from build123d import *

# Parameters (mm, degrees)
SKETCH1_R            = 7
BOSS_EXTRUDE1_DEPTH  = 8.9
CUT_EXTRUDE1_REACH   = 42.255
SKETCH6_R            = 1.3
CIRPATTERN1_COUNT    = 4
CUT_EXTRUDE2_REACH   = 42.255
SKETCH7_R            = 1.3
CUT_EXTRUDE3_DEPTH   = 5
SKETCH10_W           = 10
SKETCH10_H           = 8.9
BOSS_EXTRUDE2_DEPTH  = 10
SKETCH11_W           = 10
SKETCH11_H           = 10
BOSS_EXTRUDE3_DEPTH  = 20.4
SKETCH12_W           = 7.6
SKETCH12_H           = 7.6
CUT_EXTRUDE4_DEPTH   = 5
CUT_EXTRUDE5_REACH   = 54.931
SKETCH13_R           = 1.7
FILLET1_R            = 1
FILLET1_OF_MIRROR2_R = 1
MIRROR3_START        = -20.4
MIRROR3_OUTLINE_R    = 1.7
MIRROR3_DEPTH        = 24.3
MIRROR3_START_2      = 3.9
MIRROR3_2_DEPTH      = 5
FILLET2_R            = 0.5


# Read off the part's stored shape, not the designer's step: Mirror3
with BuildPart() as part:
    # Sketch1 → Boss-Extrude1 (new body)
    with BuildSketch(Plane(origin=(0, 0, 0), x_dir=(1, 0, 0), z_dir=(0, 1, 0))):
        with BuildLine():
            Line((-25, -28.5), (17, -28.5))
            ThreePointArc((17, -28.5), (18.414213562, -27.914213562), (19, -26.5))
            Line((19, -26.5), (19, 26.5))
            ThreePointArc((19, 26.5), (18.414213562, 27.914213562), (17, 28.5))
            Line((17, 28.5), (-25, 28.5))
            ThreePointArc((-25, 28.5), (-26.414213562, 27.914213562), (-27, 26.5))
            Line((-27, 26.5), (-27, -26.5))
            ThreePointArc((-27, -26.5), (-26.414213562, -27.914213562), (-25, -28.5))
        make_face()
        with Locations(Location((0, 0, 0), (0, 0, 270))):
            Circle(SKETCH1_R, mode=Mode.SUBTRACT)
    extrude(amount=BOSS_EXTRUDE1_DEPTH)

    # Sketch6 → Cut-Extrude1 (cut, up to next)
    with BuildSketch(Plane(origin=(0, 8.9, 0), x_dir=(1, 0, 0), z_dir=(0, 1, 0)), mode=Mode.PRIVATE) as cut_extrude1_sk1:
        with Locations(Location((-6.703372286, -6.703372286, 0), (0, 0, 270))):
            Circle(SKETCH6_R)
    cut_extrude1_tool1 = extrude(cut_extrude1_sk1.sketch, amount=-CUT_EXTRUDE1_REACH, mode=Mode.PRIVATE) & part.part
    cut_extrude1 = cut_extrude1_tool1.solids().sort_by_distance((-6.703372, 8.9, 6.703372))[0]
    add(cut_extrude1, mode=Mode.SUBTRACT)

    # CirPattern1: Cut-Extrude1 ×4 about axis
    cirpattern1_axis = Axis((0, 0, 0), (0, 1, 0))
    for i in range(1, CIRPATTERN1_COUNT):
        add(cut_extrude1.rotate(cirpattern1_axis, i * 360 / CIRPATTERN1_COUNT), mode=Mode.SUBTRACT)

    # Sketch7 → Cut-Extrude2 (cut, up to next)
    with BuildSketch(Plane(origin=(0, 8.9, 0), x_dir=(1, 0, 0), z_dir=(0, 1, 0)), mode=Mode.PRIVATE) as cut_extrude2_sk1:
        with Locations(Location((-23.5, -20, 0), (0, 0, 270))):
            Circle(SKETCH7_R)
    cut_extrude2_tool1 = extrude(cut_extrude2_sk1.sketch, amount=-CUT_EXTRUDE2_REACH, mode=Mode.PRIVATE) & part.part
    # Sketch7 → Cut-Extrude2 (cut, up to next)
    with BuildSketch(Plane(origin=(0, 8.9, 0), x_dir=(1, 0, 0), z_dir=(0, 1, 0)), mode=Mode.PRIVATE) as cut_extrude2_sk2:
        with Locations(Location((-23.5, 20, 0), (0, 0, 270))):
            Circle(SKETCH7_R)
    cut_extrude2_tool2 = extrude(cut_extrude2_sk2.sketch, amount=-CUT_EXTRUDE2_REACH, mode=Mode.PRIVATE) & part.part
    # Sketch7 → Cut-Extrude2 (cut, up to next)
    with BuildSketch(Plane(origin=(0, 8.9, 0), x_dir=(1, 0, 0), z_dir=(0, 1, 0)), mode=Mode.PRIVATE) as cut_extrude2_sk3:
        with Locations(Location((14.8, -20, 0), (0, 0, 270))):
            Circle(SKETCH7_R)
    cut_extrude2_tool3 = extrude(cut_extrude2_sk3.sketch, amount=-CUT_EXTRUDE2_REACH, mode=Mode.PRIVATE) & part.part
    # Sketch7 → Cut-Extrude2 (cut, up to next)
    with BuildSketch(Plane(origin=(0, 8.9, 0), x_dir=(1, 0, 0), z_dir=(0, 1, 0)), mode=Mode.PRIVATE) as cut_extrude2_sk4:
        with Locations(Location((14.8, 20, 0), (0, 0, 270))):
            Circle(SKETCH7_R)
    cut_extrude2_tool4 = extrude(cut_extrude2_sk4.sketch, amount=-CUT_EXTRUDE2_REACH, mode=Mode.PRIVATE) & part.part
    add(cut_extrude2_tool1.solids().sort_by_distance((-23.5, 8.9, 20))[0], mode=Mode.SUBTRACT)
    add(cut_extrude2_tool2.solids().sort_by_distance((-23.5, 8.9, -20))[0], mode=Mode.SUBTRACT)
    add(cut_extrude2_tool3.solids().sort_by_distance((14.8, 8.9, 20))[0], mode=Mode.SUBTRACT)
    add(cut_extrude2_tool4.solids().sort_by_distance((14.8, 8.9, -20))[0], mode=Mode.SUBTRACT)

    # Sketch8 → Cut-Extrude3 (cut)
    with BuildSketch(Plane(origin=(0, 8.9, 0), x_dir=(1, 0, 0), z_dir=(0, 1, 0))):
        Polygon((-20, -15), (-20, -22.5), (12, -22.5), (12, -15), (15, -15), (15, 15), (12, 15), (12, 22.5), (-20, 22.5), (-20, 15), (-23, 15), (-23, -15), align=None)
    extrude(amount=-CUT_EXTRUDE3_DEPTH, mode=Mode.SUBTRACT)

    # Sketch10 → Boss-Extrude2 (add)
    with BuildSketch(Plane.XY.offset(28.5)):
        with Locations((-19, 4.45)):
            Rectangle(SKETCH10_W, SKETCH10_H)
    boss_extrude2 = extrude(amount=BOSS_EXTRUDE2_DEPTH)

    # Sketch11 → Boss-Extrude3 (add)
    with BuildSketch(Plane.XZ):
        with Locations((-19, 33.5)):
            Rectangle(SKETCH11_W, SKETCH11_H)
    boss_extrude3 = extrude(amount=BOSS_EXTRUDE3_DEPTH)

    # Sketch12 → Cut-Extrude4 (cut)
    with BuildSketch(Plane(origin=(0, 8.9, 0), x_dir=(1, 0, 0), z_dir=(0, 1, 0))):
        with Locations((-19, -33.5)):
            Rectangle(SKETCH12_W, SKETCH12_H)
    cut_extrude4 = extrude(amount=-CUT_EXTRUDE4_DEPTH, mode=Mode.SUBTRACT)

    # Sketch13 → Cut-Extrude5 (cut, up to next)
    with BuildSketch(Plane(origin=(0, 3.9, 0), x_dir=(1, 0, 0), z_dir=(0, 1, 0)), mode=Mode.PRIVATE) as cut_extrude5_sk1:
        with Locations(Location((-19, -33.5, 0), (0, 0, 270))):
            Circle(SKETCH13_R)
    cut_extrude5_tool1 = extrude(cut_extrude5_sk1.sketch, amount=-CUT_EXTRUDE5_REACH, mode=Mode.PRIVATE) & part.part
    cut_extrude5 = cut_extrude5_tool1.solids().sort_by_distance((-19, 3.9, 33.5))[0]
    add(cut_extrude5, mode=Mode.SUBTRACT)

    # Fillet1
    fillet1_edges = [part.edges().sort_by_distance(p)[0] for p in [
        (-24, -5.75, 38.5),
        (-14, -5.75, 38.5),
        (-22.8, 6.4, 29.7),
        (-22.8, 6.4, 37.3),
        (-15.2, 6.4, 37.3),
        (-15.2, 6.4, 29.7),
    ]]
    fillet(fillet1_edges, radius=FILLET1_R)

    # Mirror2: Boss-Extrude2, Boss-Extrude3, Cut-Extrude4, Cut-Extrude5 across plane
    add(boss_extrude2.mirror(Plane.ZY.offset(9)))
    add(boss_extrude3.mirror(Plane.ZY.offset(9)))
    add(cut_extrude4.mirror(Plane.ZY.offset(9)), mode=Mode.SUBTRACT)
    add(cut_extrude5.mirror(Plane.ZY.offset(9)), mode=Mode.SUBTRACT)

    # Fillet1 of Mirror2
    fillet1_of_mirror2_edges = [part.edges().sort_by_distance(p)[0] for p in [
        (6, -5.75, 38.5),
        (-4, -5.75, 38.5),
        (4.8, 6.4, 29.7),
        (4.8, 6.4, 37.3),
        (-2.8, 6.4, 37.3),
        (-2.8, 6.4, 29.7),
    ]]
    fillet(fillet1_of_mirror2_edges, radius=FILLET1_OF_MIRROR2_R)

    # Mirror3 outline → Mirror3 (add)
    # profile 1 of 2: a face of its own
    with BuildSketch(Plane(origin=(0, 0, 0), x_dir=(1, 0, 0), z_dir=(0, 1, 0)).offset(MIRROR3_START)):
        with BuildLine():
            ThreePointArc((-23, 38.5), (-23.707106781, 38.207106781), (-24, 37.5))
            Line((-24, 37.5), (-24, 28.5))
            Line((-24, 28.5), (-14, 28.5))
            Line((-14, 28.5), (-14, 37.5))
            ThreePointArc((-14, 37.5), (-14.292893219, 38.207106781), (-15, 38.5))
            Line((-15, 38.5), (-23, 38.5))
        make_face()
        with Locations((-19, 33.5)):
            Circle(MIRROR3_OUTLINE_R, mode=Mode.SUBTRACT)
    # profile 2 of 2: a face of its own
    with BuildSketch(Plane(origin=(0, 0, 0), x_dir=(1, 0, 0), z_dir=(0, 1, 0)).offset(MIRROR3_START)):
        with BuildLine():
            Line((-4, 37.5), (-4, 28.5))
            Line((-4, 28.5), (6, 28.5))
            Line((6, 28.5), (6, 37.5))
            ThreePointArc((6, 37.5), (5.707106781, 38.207106781), (5, 38.5))
            Line((5, 38.5), (-3, 38.5))
            ThreePointArc((-3, 38.5), (-3.707106781, 38.207106781), (-4, 37.5))
        make_face()
        with Locations((1, 33.5)):
            Circle(MIRROR3_OUTLINE_R, mode=Mode.SUBTRACT)
    extrude(amount=MIRROR3_DEPTH)

    # Mirror3 2 outline → Mirror3 2 (add)
    # profile 1 of 2: a face of its own
    with BuildSketch(Plane(origin=(0, 0, 0), x_dir=(1, 0, 0), z_dir=(0, 1, 0)).offset(MIRROR3_START_2)):
        with BuildLine():
            ThreePointArc((-23, 38.5), (-23.707106781, 38.207106781), (-24, 37.5))
            Line((-24, 37.5), (-24, 28.5))
            Line((-24, 28.5), (-14, 28.5))
            Line((-14, 28.5), (-14, 37.5))
            ThreePointArc((-14, 37.5), (-14.292893219, 38.207106781), (-15, 38.5))
            Line((-15, 38.5), (-23, 38.5))
        make_face()
        with BuildLine():
            ThreePointArc((-21.8, 29.7), (-22.507106781, 29.992893219), (-22.8, 30.7))
            Line((-22.8, 30.7), (-22.8, 36.3))
            ThreePointArc((-22.8, 36.3), (-22.507106781, 37.007106781), (-21.8, 37.3))
            Line((-21.8, 37.3), (-16.2, 37.3))
            ThreePointArc((-16.2, 37.3), (-15.492893219, 37.007106781), (-15.2, 36.3))
            Line((-15.2, 36.3), (-15.2, 30.7))
            ThreePointArc((-15.2, 30.7), (-15.492893219, 29.992893219), (-16.2, 29.7))
            Line((-16.2, 29.7), (-21.8, 29.7))
        make_face(mode=Mode.SUBTRACT)
    # profile 2 of 2: a face of its own
    with BuildSketch(Plane(origin=(0, 0, 0), x_dir=(1, 0, 0), z_dir=(0, 1, 0)).offset(MIRROR3_START_2)):
        with BuildLine():
            Line((-4, 37.5), (-4, 28.5))
            Line((-4, 28.5), (6, 28.5))
            Line((6, 28.5), (6, 37.5))
            ThreePointArc((6, 37.5), (5.707106781, 38.207106781), (5, 38.5))
            Line((5, 38.5), (-3, 38.5))
            ThreePointArc((-3, 38.5), (-3.707106781, 38.207106781), (-4, 37.5))
        make_face()
        with BuildLine():
            Line((-2.8, 30.7), (-2.8, 36.3))
            ThreePointArc((-2.8, 36.3), (-2.507106781, 37.007106781), (-1.8, 37.3))
            Line((-1.8, 37.3), (3.8, 37.3))
            ThreePointArc((3.8, 37.3), (4.507106781, 37.007106781), (4.8, 36.3))
            Line((4.8, 36.3), (4.8, 30.7))
            ThreePointArc((4.8, 30.7), (4.507106781, 29.992893219), (3.8, 29.7))
            Line((3.8, 29.7), (-1.8, 29.7))
            ThreePointArc((-1.8, 29.7), (-2.507106781, 29.992893219), (-2.8, 30.7))
        make_face(mode=Mode.SUBTRACT)
    extrude(amount=MIRROR3_2_DEPTH)

    # Fillet2
    fillet2_edges = [part.edges().sort_by_distance(p)[0] for p in [
        (-23, 6.4, -15),
        (-20, 6.4, -15),
        (-20, 6.4, -22.5),
        (12, 6.4, -22.5),
        (12, 6.4, -15),
        (15, 6.4, -15),
        (15, 6.4, 15),
        (12, 6.4, 15),
        (12, 6.4, 22.5),
        (-20, 6.4, 22.5),
        (-20, 6.4, 15),
        (-23, 6.4, 15),
    ]]
    fillet(fillet2_edges, radius=FILLET2_R)


solid = part.part
Model file for the job. Use its own axes, mm. A direction names the side the tool comes from. Give positions to 0.01 mm unless a question says otherwise; leave off trailing zeros. Order: outer loops, then holes, each group sorted by start corner. A loop starts at its lowest first (then second) coordinate and runs counter-clockwise, first axis right, second up. Notation, with made-up numbers: (19.25, 89) - (71.25, 89) arc R13 ccw to (71.25, 113) - close; hole circle Ø3 at (45, 9). An arc over 180 degrees is marked (long way). Return JSON: item names as keys, results as strings.
1) Cut at B-B, the plane z = 20. Give the cut face in (x, y).
Geometry says:
{"outline": "(-27, 0) - (-24.8, 0) - (-24.8, 8.9) - (-27, 8.9) - close; (-22.2, 0) - (13.5, 0) - (13.5, 8.9) - (12, 8.9) - (12, 3.9) - (-20, 3.9) - (-20, 8.9) - (-22.2, 8.9) - close; (16.1, 0) - (19, 0) - (19, 8.9) - (16.1, 8.9) - close"}
2) Cut at C-C, the plane z = 0. Give the cut face in (x, y), plus the area to 3 significant figures.
Geometry says:
{"outline": "(-27, 0) - (-7, 0) - (-7, 3.9) - (-23, 3.9) - (-23, 8.9) - (-27, 8.9) - close; (7, 0) - (19, 0) - (19, 8.9) - (15, 8.9) - (15, 3.9) - (7, 3.9) - close", "area": "165 mm²"}
3) Cut at A-A, the plane y = -17.5. Give the cut face in (x, z).
Geometry says:
{"outline": "(-24, -37.5) arc R1 ccw to (-23, -38.5) - (-15, -38.5) arc R1 ccw to (-14, -37.5) - (-14, -28.5) - (-24, -28.5) - close; (-24, 28.5) - (-14, 28.5) - (-14, 37.5) arc R1 ccw to (-15, 38.5) - (-23, 38.5) arc R1 ccw to (-24, 37.5) - close; (-4, -37.5) arc R1 ccw to (-3, -38.5) - (5, -38.5) arc R1 ccw to (6, -37.5) - (6, -28.5) - (-4, -28.5) - close; (-4, 28.5) - (6, 28.5) - (6, 37.5) arc R1 ccw to (5, 38.5) - (-3, 38.5) arc R1 ccw to (-4, 37.5) - close; hole circle Ø3.4 at (-19, -33.5); hole circle Ø3.4 at (-19, 33.5); hole circle Ø3.4 at (1, -33.5); hole circle Ø3.4 at (1, 33.5)"}
4) Pull direction Z, two halves, no side cores. Call faces 6 (the flat face through (1, -20.4, 36)), 7 (the cylindrical face through (-26.4, 4.39, -27.93)), 8 (the flat face through (-20, 6, -19)): pulls with the +Z half, pulls with the -Z half, needs draft (parallel to the pull), parting line crosses it, or undercut.
Geometry says:
{"face 6": "needs draft", "face 7": "pulls with the -Z half", "face 8": "undercut"}
5) 3-axis set-ups, long thin cutter, end or side, ignore diameter. For faces 1 (the flat face through (-4, -6, 33)), 2 (the flat face through (1, 6, 29.7)), 3 (the cylindrical face through (0.49, -8.08, 35.12)), 4 (the flat face through (-4, -6, -33)), 5 (the flat face through (1, -10, 28.5)): which of +Z, -Z, +X, -X, +Y, -Y reach the whole face in a straight line?
Geometry says:
{"face 1": "+Z, +Y, -Y", "face 2": "+Y", "face 3": "+Y, -Y", "face 4": "-Z, +Y, -Y", "face 5": "+X, -X, -Y"}
6) Cut at D-D, the plane x = 1. Count the separate pieces of the cut face and the enclosed holes in it, plus the area to 3 significant figures.
Geometry says:
{"separate pieces": "4", "enclosed holes": "0", "area": "573 mm²"}
7) Probe line 1 (X direction, y = 2, z = 20); line 2 (X direction, y = -4, z = 33.5); line 3 (Z direction, x = 1, y = -4). List the from-to ranges inside material, lowest first. Write a range as from..to.
Geometry says:
{"line 1": "-27..-24.8, -22.2..13.5, 16.1..19", "line 2": "-24..-20.7, -17.3..-14, -4..-0.7, 2.7..6", "line 3": "-38.5..-35.2, -31.8..-28.5, 28.5..31.8, 35.2..38.5"}
8) Flat gauge pins, fed straight in: P1, Ø3, axis at x = -11, y = 3.5, coming from the +Z side; P2, Ø5.5, axis at x = 1, z = -33.5, coming from the +Y side; P3, Ø10, axis at x = 0.5, z = -22.5, coming from the -Y side. Where does each tip first touch, or does it go through?
Geometry says:
{"P1": "z = 28.5", "P2": "y = 3.9", "P3": "y = 0"}
